Source: CAD feature listing. Evaluate the final solid. Frame: model axes, mm. Give positions to 0.01 mm unless a question says otherwise; leave off trailing zeros. Loops run counter-clockwise (first coordinate to the right, second up) from the corner with the lowest first, then second, coordinate; pieces in that order, holes last.
from build123d import *

# Parameters (mm, degrees)
SKETCH_1_W          = 90
SKETCH_1_H          = 80
EXTRUDE_1_DEPTH     = 1.5
SKETCH_2_R          = 1.65
CUT_EXTRUDE_1_DEPTH = 3
FILLET_1_R          = 2
SKETCH_3_R          = 1.65
CUT_EXTRUDE_2_DEPTH = 3


with BuildPart() as part:
    # 草图1 → 凸台-拉伸1 (new, symmetric)
    with BuildSketch(Plane(origin=(0, 0, 0), x_dir=(1, 0, 0), z_dir=(0, 1, 0))):
        Rectangle(SKETCH_1_W, SKETCH_1_H)
    extrude(amount=EXTRUDE_1_DEPTH, both=True)

    # 草图2 → 切除-拉伸1 (cut)
    with BuildSketch(Plane(origin=(0, 1.5, 0), x_dir=(1, 0, 0), z_dir=(0, 1, 0))):
        with Locations(Location((12.5, 6, 0), (0, 0, 270))):
            Circle(SKETCH_2_R)
        with Locations(Location((-7.5, 6, 0), (0, 0, 270))):
            Circle(SKETCH_2_R)
        with Locations(Location((-7.5, -6, 0), (0, 0, 270))):
            Circle(SKETCH_2_R)
        with Locations(Location((12.5, -6, 0), (0, 0, 270))):
            Circle(SKETCH_2_R)
    extrude(amount=-CUT_EXTRUDE_1_DEPTH, mode=Mode.SUBTRACT)

    # 圆角1
    fillet_1_edges = [part.edges().sort_by_distance(p)[0] for p in [
        (45, 0, 40),
        (-45, 0, 40),
        (-45, 0, -40),
        (45, 0, -40),
    ]]
    fillet(fillet_1_edges, radius=FILLET_1_R)

    # 草图3 → 切除-拉伸2 (cut)
    with BuildSketch(Plane(origin=(0, 1.5, 0), x_dir=(1, 0, 0), z_dir=(0, 1, 0))):
        with Locations(Location((35, 32.5, 0), (0, 0, 270))):
            Circle(SKETCH_3_R)
        with Locations(Location((35, 23.5, 0), (0, 0, 270))):
            Circle(SKETCH_3_R)
        with Locations(Location((35, -23.5, 0), (0, 0, 270))):
            Circle(SKETCH_3_R)
        with Locations(Location((35, -32.5, 0), (0, 0, 270))):
            Circle(SKETCH_3_R)
    cut_extrude_2 = extrude(amount=-CUT_EXTRUDE_2_DEPTH, mode=Mode.SUBTRACT)

    # 镜向1: 切除-拉伸2 across plane
    add(cut_extrude_2.mirror(Plane(origin=(0, 0, 0), x_dir=(0, 0, 1), z_dir=(1, 0, 0))), mode=Mode.SUBTRACT)

    # 镜向1 at the second plane: 切除-拉伸2 across plane
    add(cut_extrude_2.mirror(Plane.XY), mode=Mode.SUBTRACT)


solid = part.part
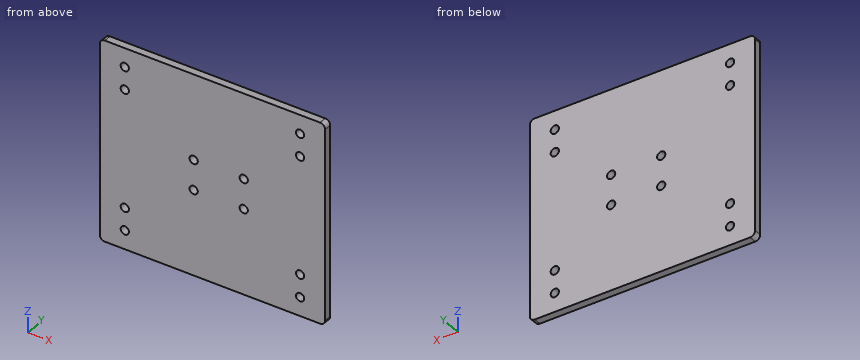
1) Cut plane C-C (x = -7.5). Return loops of the section in (y, z).
Checks:
outline: (-1.5, -40) - (1.5, -40) - (1.5, -7.65) - (-1.5, -7.65) - close; (-1.5, -4.35) - (1.5, -4.35) - (1.5, 4.35) - (-1.5, 4.35) - close; (-1.5, 7.65) - (1.5, 7.65) - (1.5, 40) - (-1.5, 40) - close
2) Cut plane B-B (x = 35). Return loops of the section in (y, z), and give its area (3 significant figures).
Checks:
outline: (-1.5, -40) - (1.5, -40) - (1.5, -34.15) - (-1.5, -34.15) - close; (-1.5, -30.85) - (1.5, -30.85) - (1.5, -25.15) - (-1.5, -25.15) - close; (-1.5, -21.85) - (1.5, -21.85) - (1.5, 21.85) - (-1.5, 21.85) - close; (-1.5, 25.15) - (1.5, 25.15) - (1.5, 30.85) - (-1.5, 30.85) - close; (-1.5, 34.15) - (1.5, 34.15) - (1.5, 40) - (-1.5, 40) - close
area: 200 mm2
3) Ray query, probe 1 along Z at (x, y) = (-35, -0.25); probe 2 along X at (y, z) = (-0.55, 23.5); probe 3 along X at (y, z) = (0.35, 6). Return the intervals inside material, ascending.
Checks:
probe 1: z = -40 to -34.15, -30.85 to -25.15, -21.85 to 21.85, 25.15 to 30.85, 34.15 to 40
probe 2: x = -45 to -36.65, -33.35 to 33.35, 36.65 to 45
probe 3: x = -45 to -9.15, -5.85 to 10.85, 14.15 to 45
4) Cut plane A-A (z = -23.5). Return loops of the section in (x, y).
Checks:
outline: (-45, -1.5) - (-36.65, -1.5) - (-36.65, 1.5) - (-45, 1.5) - close; (-33.35, -1.5) - (33.35, -1.5) - (33.35, 1.5) - (-33.35, 1.5) - close; (36.65, -1.5) - (45, -1.5) - (45, 1.5) - (36.65, 1.5) - close
5) Contact query for a flat-ended pin moving along its axis: P1, Ø5.5, axis at x = -35, z = 23.5, coming from the -Y side. Output: stop coordinate, or through.
Checks:
P1: stops at y = -1.5
